Read the model definition and answer for the solid it produces. Units are mm, in the model's axes. Give positions to 0.01 mm unless a question says otherwise; leave off trailing zeros. Write each loop counter-clockwise with the first axis right and the second up, starting at its lowest first coordinate (ties: lowest second). Pieces come first, ordered by that corner, then holes. Notation, with made-up numbers: (72, 67.5) - (93, 67.5) arc R17 ccw to (93, 84.5) - close; hole circle Ø7 at (83, -35.75). An arc over 180 degrees is marked (long way). Answer as CSV lines item,"result".
```python
from build123d import *

# Parameters (mm, degrees)
EXTRUDE_1_DEPTH     = 23
CUT_EXTRUDE_1_DEPTH = 29.235799215


with BuildPart() as part:
    # Эскиз1 → Бобышка-Вытянуть1 (new body)
    with BuildSketch(Plane(origin=(0, 0, 0), x_dir=(1, 0, 0), z_dir=(0, 1, 0))):
        with BuildLine():
            Line((-1.501479303, 16), (-3.501479303, 16))
            Line((-3.501479303, 16), (-3.501479303, -16))
            Line((-3.501479303, -16), (-1.501479303, -16))
            ThreePointArc((-1.501479303, -16), (0, 0), (-1.501479303, 16))
        make_face()
    extrude(amount=EXTRUDE_1_DEPTH)

    # Эскиз2 → Вырез-Вытянуть1 (cut, through all)
    with BuildSketch(Plane.ZY.offset(3.501479303)):
        with BuildLine():
            ThreePointArc((-10.3, 4), (-10.797918472, 5.202081528), (-12, 5.7))
            Line((-12, 5.7), (-12, 4))
            Line((-12, 4), (-10.3, 4))
        make_face()
        with BuildLine():
            Line((-12, 4), (-12, 5.7))
            ThreePointArc((-12, 5.7), (-13.202081528, 2.797918472), (-10.3, 4))
            Line((-10.3, 4), (-12, 4))
        make_face()
        with BuildLine():
            Line((-12, 17.3), (-12, 19))
            Line((-12, 19), (-10.3, 19))
            ThreePointArc((-10.3, 19), (-13.202081528, 20.202081528), (-12, 17.3))
        make_face()
        with BuildLine():
            Line((-10.3, 19), (-12, 19))
            Line((-12, 19), (-12, 17.3))
            ThreePointArc((-12, 17.3), (-10.797918472, 17.797918472), (-10.3, 19))
        make_face()
        with BuildLine():
            ThreePointArc((13.7, 19), (12, 20.7), (10.3, 19))
            Line((10.3, 19), (12, 19))
            Line((12, 19), (12, 17.3))
            ThreePointArc((12, 17.3), (13.202081528, 17.797918472), (13.7, 19))
        make_face()
        with BuildLine():
            Line((12, 19), (10.3, 19))
            ThreePointArc((10.3, 19), (10.797918472, 17.797918472), (12, 17.3))
            Line((12, 17.3), (12, 19))
        make_face()
        with BuildLine():
            ThreePointArc((13.7, 4), (13.202081528, 5.202081528), (12, 5.7))
            Line((12, 5.7), (12, 4))
            Line((12, 4), (10.3, 4))
            ThreePointArc((10.3, 4), (12, 2.3), (13.7, 4))
        make_face()
        with BuildLine():
            Line((12, 4), (12, 5.7))
            ThreePointArc((12, 5.7), (10.797918472, 5.202081528), (10.3, 4))
            Line((10.3, 4), (12, 4))
        make_face()
    extrude(amount=-CUT_EXTRUDE_1_DEPTH, mode=Mode.SUBTRACT)


solid = part.part
```
(1) A cutting plane is placed at A-A (x = -2.3). Write down the section's boundary in (y, z), and give its area (3 significant figures).
Worked out:
outline,"(0, -16) - (23, -16) - (23, 16) - (0, 16) - close; hole circle Ø3.4 at (4, -12); hole circle Ø3.4 at (4, 12); hole circle Ø3.4 at (19, -12); hole circle Ø3.4 at (19, 12)"
area,"700 mm^2"
(2) A cutting plane is placed at B-B (y = 4.75). Write down the section's boundary in (x, z), and give its area (3 significant figures).
Worked out:
outline,"(-3.5, -16) - (-1.5, -16) arc R86 ccw to (-1.07, -13.53) - (-3.5, -13.53) - close; (-3.5, -10.47) - (-0.64, -10.47) arc R86 ccw to (-0.64, 10.47) - (-3.5, 10.47) - close; (-3.5, 13.53) - (-1.07, 13.53) arc R86 ccw to (-1.5, 16) - (-3.5, 16) - close"
area,"79.9 mm^2"
(3) A cutting plane is placed at C-C (y = 10.5). Write down the section's boundary in (x, z), and give its area (3 significant figures).
Worked out:
outline,"(-3.5, -16) - (-1.5, -16) arc R86 ccw to (-1.5, 16) - (-3.5, 16) - close"
area,"96.1 mm^2"
(4) A cutting plane is placed at D-D (z = -4.5). Write down the section's boundary in (x, y), and give its area (3 significant figures).
Worked out:
outline,"(-3.5, 0) - (-0.12, 0) - (-0.12, 23) - (-3.5, 23) - close"
area,"77.8 mm^2"
(5) Find the intervals of material crossed by L1, parallel to Z at x = -2.1, y = 4; L2, parallel to Y at x = -1.45, z = -12; L3, parallel to X at y = 20, z = 0.5, in increasing order.
Worked out:
L1,"z = -16 to -13.7, -10.3 to 10.3, 13.7 to 16"
L2,"y = 0 to 2.3, 5.7 to 17.3, 20.7 to 23"
L3,"x = -3.5 to 0"
(6) Each of these flat-tipped pins is pushed along its axis until it touches: P1, Ø2.5, axis at y = 19, z = -12, coming from the -X side; P2, Ø5, axis at y = 8.5, z = -4.5, coming from the +X side. Where does it stop, or does it pass through?
Worked out:
P1,"passes through"
P2,"stops at x = -0.02"
